Here's how the part is built. I have some questions about the finished solid (model axes, mm). Give positions to 0.01 mm unless a question says otherwise; leave off trailing zeros. Loops run counter-clockwise (first coordinate to the right, second up) from the corner with the lowest first, then second, coordinate; pieces in that order, holes last.
Q1. Suppose I cut it at B-B (z = 1.75). Count the separate pieces of the cut face and the enclosed holes in it, and give its area (3 significant figures).
Q2. I'm going to push flat-ended pins straight in: P1, Ø2, axis at y = -4.5, z = 3, coming from the +X side; P2, Ø1.5, axis at y = 46.5, z = 3, coming from the +X side; P3, Ø3, axis at y = 24, z = 3.5, coming from the -X side. Where does each tip first touch, or does it pass through?
Q3. I need wall thicknesses on probe 1 along X at (y, z) = (-7, 1.75); probe 2 along Y at (x, z) = (83.25, 3); probe 3 along X at (y, z) = (24, 2). Which ranges of each line are inside material? Lowest first, please.
Q4. Suppose I cut it at A-A (y = -6.5). List the corners of the cut face in (x, z) for me, and give its area (3 significant figures).
Autodesk Inventor part; units mm, degrees
ref_plane "YZ Plane" through (0, 0, 0) normal (1, 0, 0) x (0, 1, 0)
ref_plane "XZ Plane" through (0, 0, 0) normal (0, 1, 0) x (-1, 0, 0)
ref_plane "XY Plane" through (0, 0, 0) normal (0, 0, 1) x (1, 0, 0)
sketch "Sketch1" plane through (0, 0, 0) normal (0, 0, 1) x (1, 0, 0)
  line L0 (0, 0) -> (335, 0)
  line L1 (335, 0) -> (335, 55)
  line L2 (0, 55) -> (0, 0)
  line L3 (30, 55) -> (40, 45)
  line L4 (40, 45) -> (295, 45)
  line L5 (295, 45) -> (305, 55)
  line L6 (335, 55) -> (305, 55)
  line L7 (30, 55) -> (0, 55)
  dimension "d0" = 335
  dimension "d1" = 55
  dimension "d2" = 45
  dimension "d3" = 30
  dimension "d4" = 10
  dimension "d5" = 30
extrude "Extrusion1" add sketch "Sketch1" along normal blind 6.5
sketch "Sketch2" plane through (0, 0, 6.5) normal (0, 0, 1) x (1, 0, 0)
  line L0 (0, 0) -> (335, 0)
  line L1 (295, 45) -> (40, 45)
  line L2 (0, 55) -> (0, 0)
  line L3 (0, 25.25) -> (0, 29.75)
  line L4 (16.3, 29.75) -> (16.3, 25.25)
  line L5 (5, 32.25) -> (12.3, 32.25)
  line L6 (12.3, 22.75) -> (5, 22.75)
  line L7 (0, 29.75) -> (5, 29.75)
  line L8 (12.3, 29.75) -> (16.3, 29.75)
  line L9 (16.3, 25.25) -> (12.3, 25.25)
  line L10 (5, 25.25) -> (0, 25.25)
  line L11 (5, 22.75) -> (5, 25.25)
  line L12 (5, 29.75) -> (5, 32.25)
  line L13 (12.3, 32.25) -> (12.3, 29.75)
  line L14 (12.3, 25.25) -> (12.3, 22.75)
  line L15 (167.5, 0) -> (167.5, 45) construction
  line L16 (335, 25.25) -> (335, 29.75)
  line L17 (318.7, 29.75) -> (318.7, 25.25)
  line L18 (330, 32.25) -> (322.7, 32.25)
  line L19 (322.7, 22.75) -> (330, 22.75)
  line L20 (335, 29.75) -> (330, 29.75)
  line L21 (322.7, 29.75) -> (318.7, 29.75)
  line L22 (318.7, 25.25) -> (322.7, 25.25)
  line L23 (330, 25.25) -> (335, 25.25)
  line L24 (330, 22.75) -> (330, 25.25)
  line L25 (330, 29.75) -> (330, 32.25)
  line L26 (322.7, 32.25) -> (322.7, 29.75)
  line L27 (322.7, 25.25) -> (322.7, 22.75)
  point P0 (0, 27.5)
  point P1 (0, 27.5)
  point P2 (335, 27.5)
  point P3 (335, 27.5)
  dimension "d8" = 4.5
  dimension "d9" = 2.5
  dimension "d10" = 2.5
  dimension "d11" = 5
  dimension "d12" = 7.3
  dimension "d13" = 4
extrude "Extrusion2" cut sketch "Sketch2" against normal through all
sketch "Sketch3" plane through (0, 0, 6.5) normal (0, 0, 1) x (1, 0, 0)
  line L0 (0, 25.25) -> (0, 0)
  line L1 (0, 0) -> (335, 0)
  line L2 (335, 0) -> (335, 25.25)
  line L3 (335, 29.75) -> (335, 55)
  line L4 (0, 55) -> (0, 29.75)
  line L5 (16.3, 29.75) -> (16.3, 25.25)
  line L6 (0, 43) -> (-4.5, 43)
  line L7 (-6.5, 41) -> (-6.5, 37)
  line L8 (-4.5, 35) -> (0, 35)
  line L9 (0, 35) -> (0, 43)
  line L10 (0, 20) -> (-4.5, 20)
  line L11 (-6.5, 18) -> (-6.5, 14)
  line L12 (-4.5, 12) -> (0, 12)
  line L13 (0, 12) -> (0, 20)
  arc A0 (-4.5, 43) -> (-6.5, 41) centre (-4.5, 41) ccw
  arc A1 (-6.5, 37) -> (-4.5, 35) centre (-4.5, 37) ccw
  arc A2 (-4.5, 20) -> (-6.5, 18) centre (-4.5, 18) ccw
  arc A3 (-6.5, 14) -> (-4.5, 12) centre (-4.5, 14) ccw
  line L14 (335, 43) -> (339.5, 43)
  line L15 (341.5, 41) -> (341.5, 37)
  line L16 (339.5, 35) -> (335, 35)
  line L17 (335, 35) -> (335, 43)
  line L18 (335, 20) -> (339.5, 20)
  line L19 (341.5, 18) -> (341.5, 14)
  line L20 (339.5, 12) -> (335, 12)
  line L21 (335, 12) -> (335, 20)
  arc A4 (341.5, 41) -> (339.5, 43) centre (339.5, 41) ccw
  arc A5 (339.5, 35) -> (341.5, 37) centre (339.5, 37) ccw
  arc A6 (341.5, 18) -> (339.5, 20) centre (339.5, 18) ccw
  arc A7 (339.5, 12) -> (341.5, 14) centre (339.5, 14) ccw
  line L22 (197.8, 0) -> (205.8, 0)
  line L23 (205.8, 0) -> (205.8, -11)
  line L24 (203.8, -13) -> (199.8, -13)
  line L25 (197.8, -11) -> (197.8, 0)
  line L26 (137.2, 0) -> (129.2, 0)
  line L27 (129.2, 0) -> (129.2, -11)
  line L28 (131.2, -13) -> (135.2, -13)
  line L29 (137.2, -11) -> (137.2, 0)
  line L30 (60.6, 0) -> (68.6, 0)
  line L31 (68.6, 0) -> (68.6, -11)
  line L32 (66.6, -13) -> (62.6, -13)
  line L33 (60.6, -11) -> (60.6, 0)
  line L34 (266.4, 0) -> (274.4, 0)
  line L35 (274.4, 0) -> (274.4, -11)
  line L36 (272.4, -13) -> (268.4, -13)
  line L37 (266.4, -11) -> (266.4, 0)
  arc A8 (60.6, -11) -> (62.6, -13) centre (62.6, -11) ccw
  arc A9 (66.6, -13) -> (68.6, -11) centre (66.6, -11) ccw
  arc A10 (129.2, -11) -> (131.2, -13) centre (131.2, -11) ccw
  arc A11 (135.2, -13) -> (137.2, -11) centre (135.2, -11) ccw
  arc A12 (197.8, -11) -> (199.8, -13) centre (199.8, -11) ccw
  arc A13 (203.8, -13) -> (205.8, -11) centre (203.8, -11) ccw
  arc A14 (266.4, -11) -> (268.4, -13) centre (268.4, -11) ccw
  arc A15 (272.4, -13) -> (274.4, -11) centre (272.4, -11) ccw
  line L38 (68.6, -5.5) -> (129.2, -5.5) construction
  line L39 (137.2, -5.5) -> (197.8, -5.5) construction
  line L40 (205.8, -5.5) -> (266.4, -5.5) construction
  line L41 (274.4, -5.5) -> (335, -5.5) construction
  line L42 (60.6, -5.5) -> (0, -5.5) construction
  point P0 (16.3, 27.5)
  point P1 (167.5, 0)
  dimension "d16" = 2
  dimension "d17" = 8
  dimension "d18" = 8
  dimension "d19" = 15
  dimension "d20" = 7.5
  dimension "d21" = 6.5
  dimension "d22" = 2
  dimension "d23" = 6.5
  dimension "d24" = 2
  dimension "d25" = 8
  dimension "d26" = 8
  dimension "d27" = 8
  dimension "d28" = 8
  dimension "d29" = 13
extrude "Extrusion3" add sketch "Sketch3" against normal blind 6.5
sketch "Sketch4" plane through (0, 0, 6.5) normal (0, 0, 1) x (1, 0, 0)
  line L0 (0, 20) -> (-4.5, 20)
  arc A0 (-4.5, 20) -> (-6.5, 18) centre (-4.5, 18) ccw
  line L1 (-6.5, 18) -> (-6.5, 14)
  arc A1 (-6.5, 14) -> (-4.5, 12) centre (-4.5, 14) ccw
  line L2 (-4.5, 12) -> (0, 12)
  line L3 (335, 12) -> (339.5, 12)
  arc A2 (339.5, 12) -> (341.5, 14) centre (339.5, 14) ccw
  line L4 (341.5, 14) -> (341.5, 18)
  arc A3 (341.5, 18) -> (339.5, 20) centre (339.5, 18) ccw
  line L5 (339.5, 20) -> (335, 20)
  line L6 (5, 22.75) -> (5, 25.25)
  line L7 (0, 20) -> (0, 12)
  line L8 (335, 20) -> (335, 12)
extrude "Extrusion4" cut sketch "Sketch4" against normal through all
sketch "Sketch5" plane through (0, 0, 6.5) normal (0, 0, 1) x (1, 0, 0)
  line L0 (0, 25.25) -> (0, 0)
  line L1 (0, 0) -> (60.6, 0)
  line L2 (335, 0) -> (335, 25.25)
  circle A0 centre (83.25, 20) radius 2.25
  circle A1 centre (251.75, 20) radius 2.25
  dimension "d34" = 4.5
  dimension "d35" = 20
  dimension "d36" = 83.25
  dimension "d37" = 83.25
extrude "Extrusion5" cut sketch "Sketch5" against normal through all
equation "\"d5\" = d3"
equation "\"d23\" = d21"
equation "\"d37\" = d36"
properties part number "frame_brace_top"
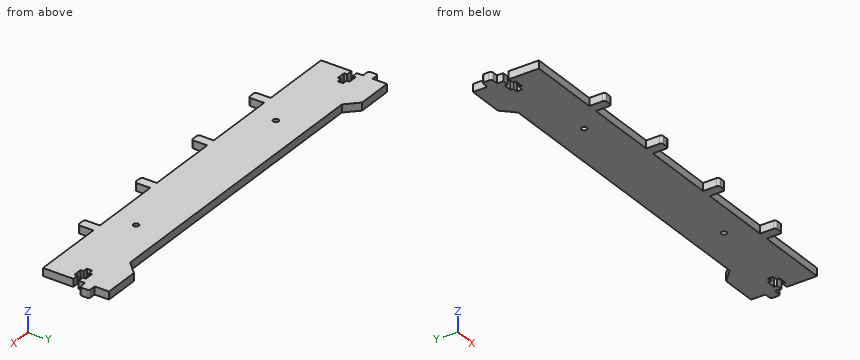
Solutions:
1. separate pieces: 1
1. enclosed holes: 2
1. area: 16,000 mm2
2. P1: stops at x = 274.4
2. P2: stops at x = 335
2. P3: stops at x = 0
3. probe 1: x = 60.6 to 68.6, 129.2 to 137.2, 197.8 to 205.8, 266.4 to 274.4
3. probe 2: y = 0 to 17.75, 22.25 to 45
3. probe 3: x = 0 to 5, 12.3 to 322.7, 330 to 335
4. outline: (60.6, 0) - (68.6, 0) - (68.6, 6.5) - (60.6, 6.5) - close; (129.2, 0) - (137.2, 0) - (137.2, 6.5) - (129.2, 6.5) - close; (197.8, 0) - (205.8, 0) - (205.8, 6.5) - (197.8, 6.5) - close; (266.4, 0) - (274.4, 0) - (274.4, 6.5) - (266.4, 6.5) - close
4. area: 208 mm2
